from build123d import *

# Parameters (mm, degrees)
SKETCH1_W               = 101.6
SKETCH1_H               = 107.95
BOSS_EXTRUDE1_DEPTH     = 3.175
CUT_EXTRUDE1_DEPTH      = 75.189091179
CUT_EXTRUDE1_DEPTH_BACK = 75.189091179
SKETCH2_W               = 3.429
SKETCH2_H               = 6.604
SKETCH3_W               = 101.6
SKETCH3_H               = 50.8
CUT_EXTRUDE2_DEPTH      = 75.189091179


with BuildPart() as part:
    # Sketch1 → Boss-Extrude1 (new body)
    with BuildSketch(Plane(origin=(0, 0, 0), x_dir=(1, 0, 0), z_dir=(0, 1, 0))):
        Rectangle(SKETCH1_W, SKETCH1_H)
    extrude(amount=BOSS_EXTRUDE1_DEPTH)

    # Sketch2 → Cut-Extrude1 (cut, two sides: drawn at the far end of the back side and taken through both)
    with BuildSketch(Plane(origin=(0, 3.175, 0), x_dir=(1, 0, 0), z_dir=(0, 1, 0)).offset(-CUT_EXTRUDE1_DEPTH_BACK)):
        Polygon((22.098, -47.625), (28.194, -47.625), (28.194, -54.229), (34.798, -54.229), (34.798, -47.625), (47.371, -47.625), (47.371, -41.021), (50.8, -41.021), (50.8, -47.625), (50.8, -92.544961432), (-50.8, -92.544961432), (-50.8, -47.625), (-50.8, -41.021), (-47.371, -41.021), (-47.371, -47.625), (-35.306, -47.625), (-35.306, -54.229), (-28.702, -54.229), (-28.702, -47.625), (-22.606, -47.625), (-22.606, -54.229), (-16.002, -54.229), (-16.002, -47.625), (-9.906, -47.625), (-9.906, -54.229), (-3.302, -54.229), (-3.302, -47.625), (2.794, -47.625), (2.794, -54.229), (9.398, -54.229), (9.398, -47.625), (15.494, -47.625), (15.494, -54.229), (22.098, -54.229), align=None)
        with Locations((-49.0855, 31.75)):
            Rectangle(SKETCH2_W, SKETCH2_H)
        with Locations((-49.0855, 19.177)):
            Rectangle(SKETCH2_W, SKETCH2_H)
        with Locations((-49.0855, 6.477)):
            Rectangle(SKETCH2_W, SKETCH2_H)
        with Locations((-49.0855, -6.223)):
            Rectangle(SKETCH2_W, SKETCH2_H)
        with Locations((-49.0855, -18.923)):
            Rectangle(SKETCH2_W, SKETCH2_H)
        with Locations((-49.0855, -31.623)):
            Rectangle(SKETCH2_W, SKETCH2_H)
        with Locations((49.0855, -31.623)):
            Rectangle(SKETCH2_W, SKETCH2_H)
        with Locations((49.0855, -18.923)):
            Rectangle(SKETCH2_W, SKETCH2_H)
        with Locations((49.0855, -6.223)):
            Rectangle(SKETCH2_W, SKETCH2_H)
        with Locations((49.0855, 6.477)):
            Rectangle(SKETCH2_W, SKETCH2_H)
        with Locations((49.0855, 19.177)):
            Rectangle(SKETCH2_W, SKETCH2_H)
        with Locations((49.0855, 31.75)):
            Rectangle(SKETCH2_W, SKETCH2_H)
        with Locations((49.0855, 44.45)):
            Rectangle(SKETCH2_W, SKETCH2_H)
        with Locations((-49.0855, 44.45)):
            Rectangle(SKETCH2_W, SKETCH2_H)
    extrude(amount=CUT_EXTRUDE1_DEPTH + CUT_EXTRUDE1_DEPTH_BACK, mode=Mode.SUBTRACT)

    # Sketch3 → Cut-Extrude2 (cut, through all)
    with BuildSketch(Plane(origin=(0, 3.175, 0), x_dir=(1, 0, 0), z_dir=(0, 1, 0))):
        with Locations((0, 28.575)):
            Rectangle(SKETCH3_W, SKETCH3_H)
    extrude(amount=-CUT_EXTRUDE2_DEPTH, mode=Mode.SUBTRACT)


solid = part.part
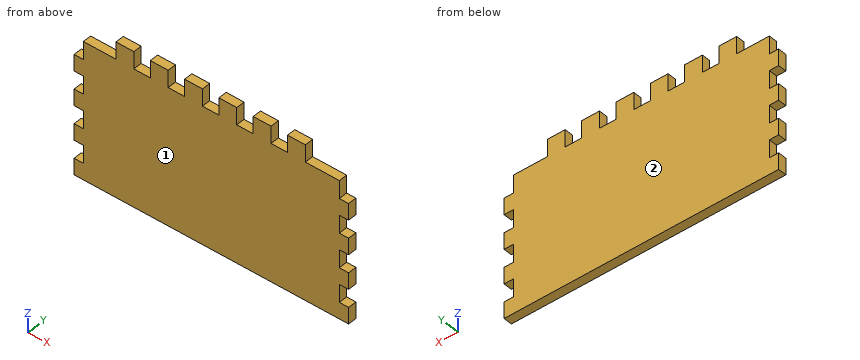
Could you check a few things on this model? Use its own coordinates, in mm. Face numbers are marked on the shaded views. Give positions to 0.01 mm unless a question says otherwise; leave off trailing zeros. Order: outer loops, then holes, each group sorted by start corner. A loop starts at its lowest first (then second) coordinate and runs counter-clockwise, first axis right, second up.
1. Suppose I cut it at A-A (z = 50). List the corners of the cut face in (x, y) for me (3 decimals), plus the area to 3 significant figures.
2. We'd pull the mould along Y, two halves only. Please class the marked faces 1 and 2: pulls with the +Y half, pulls with the -Y half, needs draft (parallel to the pull), parting line crosses it, or undercut.
3. Will these pins go through, and if not, where does the flat tip stop? P1, Ø1.6, axis at y = 2, z = 49.5, coming from the -X side; P2, Ø1.6, axis at y = 1.5, z = 33, coming from the +X side; P3, Ø1.6, axis at x = 50, y = 1.5, coming from the +Z side.
4. Suppose I cut it at C-C (z = 8). List the corners of the cut face in (x, y) for me (3 decimals).
5. I need wall thicknesses on L1, parallel to X at y = 1.45, z = 50.5; L2, parallel to X at y = 1.2, z = 20; L3, parallel to Z at x = -47, y = 0.8 (3 decimals). Which ranges of each line are inside material? Lowest first, please.
6. Suppose I cut it at B-B (x = 43.5). List the corners of the cut face in (y, z) for me (3 decimals), plus the area to 3 significant figures.
Solved:
1. outline: (-35.306, 0) - (-28.702, 0) - (-28.702, 3.175) - (-35.306, 3.175) - close; (-22.606, 0) - (-16.002, 0) - (-16.002, 3.175) - (-22.606, 3.175) - close; (-9.906, 0) - (-3.302, 0) - (-3.302, 3.175) - (-9.906, 3.175) - close; (2.794, 0) - (9.398, 0) - (9.398, 3.175) - (2.794, 3.175) - close; (15.494, 0) - (22.098, 0) - (22.098, 3.175) - (15.494, 3.175) - close; (28.194, 0) - (34.798, 0) - (34.798, 3.175) - (28.194, 3.175) - close
1. area: 126 mm2
2. face 1: pulls with the -Y half
2. face 2: pulls with the +Y half
3. P1: stops at x = -35.31
3. P2: stops at x = 47.37
3. P3: stops at z = 41.02
4. outline: (-47.371, 0) - (47.371, 0) - (47.371, 3.175) - (-47.371, 3.175) - close
5. L1: x = -35.31 to -28.7, -22.61 to -16, -9.91 to -3.3, 2.79 to 9.4, 15.49 to 22.1, 28.19 to 34.8
5. L2: x = -47.37 to 47.37
5. L3: z = -3.175 to 47.625
6. outline: (0, -3.175) - (3.175, -3.175) - (3.175, 47.625) - (0, 47.625) - close
6. area: 161 mm2
